from build123d import *

# Parameters (mm, degrees)
SKETCH_1_W           = 30
SKETCH_1_H           = 30
EXTRUDE_1_DEPTH      = 30
SKETCH_42_W          = 10
SKETCH_42_H          = 10
CUT_EXTRUDE_29_DEPTH = 52.961524227
SKETCH_43_W          = 20
SKETCH_43_H          = 10
CUT_EXTRUDE_30_DEPTH = 52.961524227
SKETCH_44_W          = 10
SKETCH_44_H          = 10
CUT_EXTRUDE_31_DEPTH = 47.904157598


with BuildPart() as part:
    # 草圖1 → 填料-伸1 (new body)
    with BuildSketch(Plane.XY):
        with Locations((15, 15)):
            Rectangle(SKETCH_1_W, SKETCH_1_H)
    extrude(amount=-EXTRUDE_1_DEPTH)

    # 草圖42 → 除料-伸長29 (cut, through all)
    with BuildSketch(Plane.XY):
        with Locations((15, 25)):
            Rectangle(SKETCH_42_W, SKETCH_42_H)
    extrude(amount=-CUT_EXTRUDE_29_DEPTH, mode=Mode.SUBTRACT)

    # 草圖43 → 除料-伸長30 (cut, through all)
    with BuildSketch(Plane(origin=(30, 0, 0), x_dir=(0, 0, -1), z_dir=(1, 0, 0))):
        Polygon((30, 30), (20, 30), (20, 20), align=None)
        with Locations((10, 25)):
            Rectangle(SKETCH_43_W, SKETCH_43_H)
    extrude(amount=-CUT_EXTRUDE_30_DEPTH, mode=Mode.SUBTRACT)

    # 草圖44 → 除料-伸長31 (cut, through all)
    with BuildSketch(Plane(origin=(0, 20, 0), x_dir=(1, 0, 0), z_dir=(0, 1, 0))):
        with Locations((15, 5)):
            Rectangle(SKETCH_44_W, SKETCH_44_H)
    extrude(amount=-CUT_EXTRUDE_31_DEPTH, mode=Mode.SUBTRACT)


solid = part.part
For this review, take the finished solid that the model builds, in its own axes (mm). A direction names the side the tool comes from. Give positions to 0.01 mm unless a question says otherwise; leave off trailing zeros. Loops run counter-clockwise (first coordinate to the right, second up) from the corner with the lowest first, then second, coordinate; pieces in that order, holes last.
Item 1: Insertion check: pin 1 (1.5 mm diameter, centred on x = 20.5, z = -9.5, fed in from -Y); pin 2 (5 mm diameter, centred on x = 13, y = 8.5, fed in from +Z); pin 3 (1.5 mm diameter, centred on x = 22, z = -11.5, fed in from +Y). Each pin has a flat end and moves straight along its axis. Give the tip position at first contact, or say it passes through.
Item 2: Take a section at D-D, the plane y = 19. State the section outline as (x, z) points.
Item 3: Draft analysis for pull direction X (two halves, no side actions). For faces 6 (the flat face through (25, 10, 0)), 7 (the flat face through (0, 11, -15)), 8 (the flat face through (20, 10, -5)), state which applies: +X half, -X half, draft (parallel to the pull), parting line (faces both ways), or undercut.
Item 4: Take a section at A-A, the plane y = 22.5. State the section outline as (x, z) points, and give its area (3 significant figures).
Item 5: Take a section at C-C, the plane z = -20.5. State the section outline as (x, y) points, and give its area (3 significant figures).
Item 6: Take a section at B-B, the plane z = -2. State the section outline as (x, y) points.
Item 7: Tool access review of faces 1 (the flat face through (15, 0, -15)), 2 (the flat face through (10, 10, -5)), 3 (the flat face through (20, 23, -27)), 4 (the flat face through (25, 25, -25)), 5 (the flat face through (15, 20, -15)): name each direction out of +Z, -Z, +X, -X, +Y, -Y from which nothing blocks a thin tool from reaching the whole face with its end or side.
Item 8: For line 1 along X through (y, z) = (23, -27.5); line 2 along Y through (x, z) = (19.5, -12); line 3 along Z through (x, y) = (23, 21.5), list the stretches that pass through material, from the lowest coordinate up.
Calculated:
1. pin 1: stops at y = 0
1. pin 2: stops at z = -10
1. pin 3: stops at y = 20
2. outline: (0, -30) - (30, -30) - (30, 0) - (20, 0) - (20, -10) - (10, -10) - (10, 0) - (0, 0) - close
3. face 6: draft
3. face 7: -X half
3. face 8: undercut
4. outline: (0, -30) - (10, -30) - (10, -22.5) - (0, -22.5) - close; (20, -30) - (30, -30) - (30, -22.5) - (20, -22.5) - close
4. area: 150 mm2
5. outline: (0, 0) - (30, 0) - (30, 20.5) - (20, 20.5) - (20, 20) - (10, 20) - (10, 20.5) - (0, 20.5) - close
5. area: 610 mm2
6. outline: (0, 0) - (10, 0) - (10, 20) - (0, 20) - close; (20, 0) - (30, 0) - (30, 20) - (20, 20) - close
7. face 1: +Z, -Z, +X, -X, -Y
7. face 2: +Z, +Y, -Y
7. face 3: +Z, -Z, +Y
7. face 4: +Z, +X, -X, +Y
7. face 5: +Z, +Y
8. line 1: x = 0 to 10, 20 to 30
8. line 2: y = 0 to 20
8. line 3: z = -30 to -21.5
